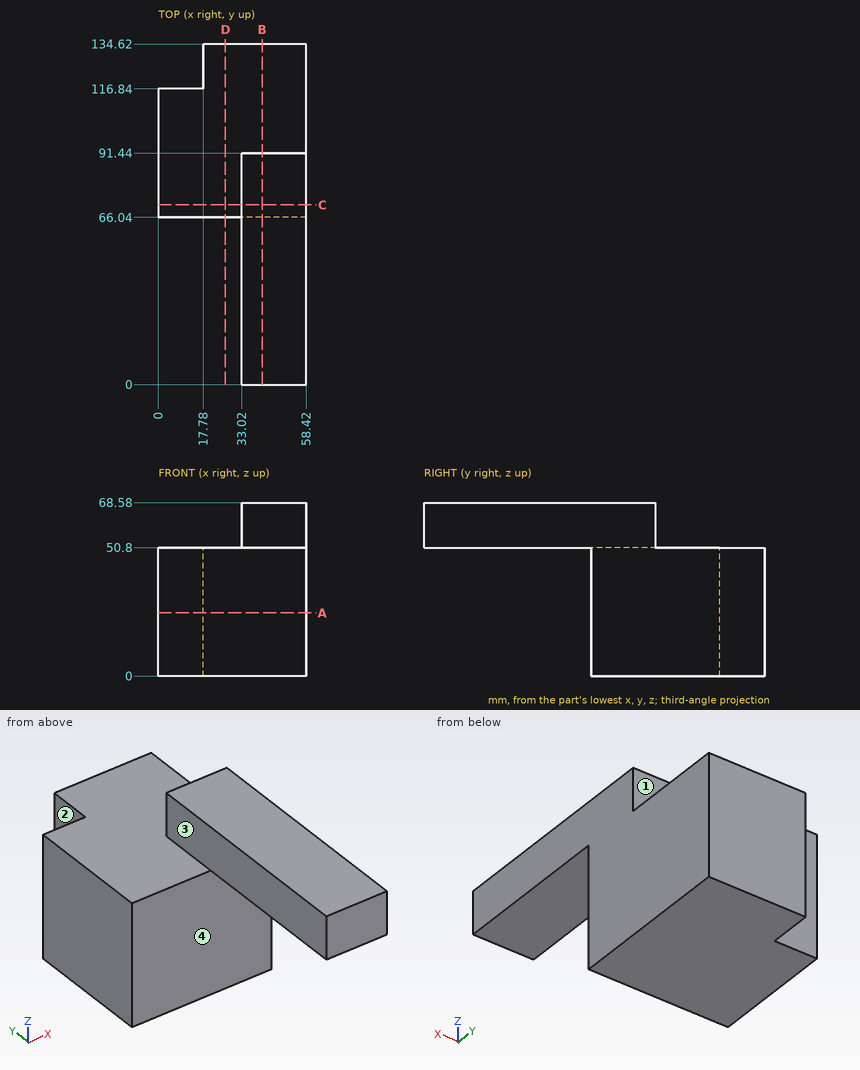
Part print with two shaded views. Sizes in mm from the minimum x, y, z corner. A direction names the side the tool comes from. Coordinates: 2 decimals unless noted, no trailing zeros. Loops run counter-clockwise (first coordinate to the right, second up) from the corner with the lowest first, then second, coordinate; pieces in that order, holes last. Notation, with made-up numbers: (15.25, -34) - (26.25, -34) arc R23 cw to (26.25, 0) - close; hole circle Ø1 at (8.25, 79). An arc over 180 degrees is marked (long way). Write each question's results on one line, items separated by ' | '. Start each with the question number.
Q1. Slice it at D-D on x = 26.5. Give the cut face in (y, z).
Q2. Which spindle directions (+Z, -Z, +X, -X, +Y, -Y) get a long thin tool onto all of the face, cutting with end or side? Do the marked faces 1, 2, 3 and 4. Say none if no direction does.
Q3. Drop flat-ended pins along their axis: pin 1 Ø14 at (y, z) = (31, 57.5) entering from -X; pin 2 Ø14 at (x, z) = (47.5, 63) entering from +Y; pin 3 Ø6 at (x, z) = (29.5, 14) entering from -Y. Give the stop position or say it passes through.
Q4. Slice it at C-C on y = 71. Give the cut face in (x, z), and give its area (3 significant figures).
Q5. Slice it at B-B on x = 41. Give the cut face in (y, z).
Q6. Slice it at A-A on z = 25. Give the cut face in (x, y).
Q7. Probe line 1 along Z through (x, y) = (42, 37.5); line 2 along Y through (x, z) = (30, 20); line 3 along Z through (x, y) = (39.5, 120). List the from-to ranges inside material, lowest first.
Answer:
1) outline: (66.04, 0) - (134.62, 0) - (134.62, 50.8) - (66.04, 50.8) - close
2) face 1: +Z, +X, -X, +Y | face 2: +Z, -Z, -X, +Y | face 3: +Z, -X, +Y, -Y | face 4: -Z, +X, -X, -Y
3) pin 1: stops at x = 33.02 | pin 2: stops at y = 91.44 | pin 3: stops at y = 66.04
4) outline: (0, 0) - (58.42, 0) - (58.42, 68.58) - (33.02, 68.58) - (33.02, 50.8) - (0, 50.8) - close | area: 3,420 mm2
5) outline: (0, 50.8) - (66.04, 50.8) - (66.04, 0) - (134.62, 0) - (134.62, 50.8) - (91.44, 50.8) - (91.44, 68.58) - (0, 68.58) - close
6) outline: (0, 66.04) - (58.42, 66.04) - (58.42, 134.62) - (17.78, 134.62) - (17.78, 116.84) - (0, 116.84) - close
7) line 1: z = 50.8 to 68.58 | line 2: y = 66.04 to 134.62 | line 3: z = 0 to 50.8
